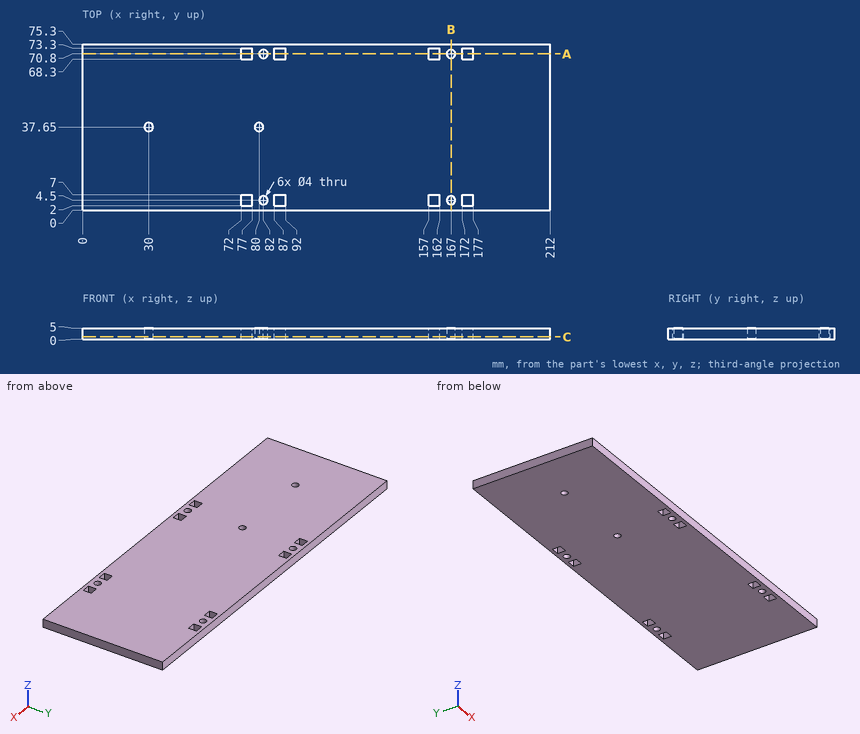
Verification items for this drawing (mm, ordinates from the low corner). Round coordinates to 2 decimals unless told otherwise and drop trailing zeros. Order: outer loops, then holes, each group sorted by start corner. A loop starts at its lowest first (then second) coordinate and runs counter-clockwise, first axis right, second up. Notation, with made-up numbers: M 55,59 L 89,59 A21 ccw 89,80 Z; hole C 16,27.5 d6. An arc over 180 degrees is marked long. Answer in a Markdown table with one row per item. Add a question column.
Item 1: Sectioned sample at B-B, the plane x = 167. Enter the section's corners in (y, z).
Item 2: Sectioned sample at C-C, the plane z = 1.05. State how many separate pieces and enclosed holes the cut face has, plus the area to 3 significant figures.
Item 3: Sectioned sample at A-A, the plane y = 70.8. Enter the section's corners in (x, z).
Item 4: Material ranges on L1, parallel to Y at x = 76.5, z = 1.95; L2, parallel to Y at x = 30, z = 2, recorded low to high. Write a range as [from, to].
Filled in:
| question | item | result |
|---|---|---|
| 1 | outline | M 0,0 L 2.5,0 L 2.5,5 L 0,5 Z; M 6.5,0 L 68.8,0 L 68.8,5 L 6.5,5 Z; M 72.8,0 L 75.3,0 L 75.3,5 L 72.8,5 Z |
| 2 | separate pieces | 1 |
| 2 | enclosed holes | 14 |
| 2 | area | 15,700 mm² |
| 3 | outline | M 0,0 L 72,0 L 72,5 L 0,5 Z; M 77,0 L 80,0 L 80,5 L 77,5 Z; M 84,0 L 87,0 L 87,5 L 84,5 Z; M 92,0 L 157,0 L 157,5 L 92,5 Z; M 162,0 L 165,0 L 165,5 L 162,5 Z; M 169,0 L 172,0 L 172,5 L 169,5 Z; M 177,0 L 212,0 L 212,5 L 177,5 Z |
| 4 | L1 | y = [0, 2], [7, 68.3], [73.3, 75.3] |
| 4 | L2 | y = [0, 35.65], [39.65, 75.3] |
